from build123d import *

# Parameters (mm, degrees)
SKETCH1_W           = 20
SKETCH1_H           = 20
BOSS_EXTRUDE1_DEPTH = 20
SKETCH2_W           = 45
SKETCH2_H           = 70
BOSS_EXTRUDE2_DEPTH = 9
CUT_EXTRUDE1_DEPTH  = 5.8
FILLET1_R           = 3.6
FILLET2_R           = 10
SKETCH5_R           = 3.9
CUT_EXTRUDE2_DEPTH  = 51.717354032
CUT_EXTRUDE3_REACH  = 49.639
SKETCH6_R           = 1.75
SKETCH7_W           = 9
SKETCH7_H           = 45
CUT_EXTRUDE4_DEPTH  = 4.8
SKETCH9_W           = 9
SKETCH9_H           = 45
CUT_EXTRUDE5_DEPTH  = 23.8
SKETCH10_W          = 12.5
SKETCH10_H          = 41.4
CUT_EXTRUDE6_DEPTH  = 23.8
SKETCH11_W          = 20
SKETCH11_H          = 1.2
CUT_EXTRUDE7_DEPTH  = 23.8
BOSS_EXTRUDE3_START = 20
SKETCH12_W          = 20
SKETCH12_H          = 20
SKETCH12_R          = 3.9
BOSS_EXTRUDE3_DEPTH = 20
SKETCH13_W          = 20.2
SKETCH13_H          = 20.2
SKETCH13_R          = 3.9
BOSS_EXTRUDE4_DEPTH = 40
SKETCH14_W          = 9
SKETCH14_H          = 20
BOSS_EXTRUDE5_DEPTH = 0.1
SKETCH15_W          = 9
SKETCH15_H          = 40.3
BOSS_EXTRUDE6_DEPTH = 0.1
SKETCH16_W          = 9
SKETCH16_H          = 40.3
BOSS_EXTRUDE7_DEPTH = 0.1
SKETCH17_R          = 4.83091966
BOSS_EXTRUDE8_DEPTH = 39
SKETCH18_R          = 3
CUT_EXTRUDE8_DEPTH  = 2
FILLET3_R           = 3.23
FILLET4_R           = 4


# Some blends are built 0.0001 mm under size
with BuildPart() as part:
    # Sketch1 → Boss-Extrude1 (new body)
    with BuildSketch(Plane(origin=(0, 0, 0), x_dir=(0, 0, -1), z_dir=(1, 0, 0))):
        Rectangle(SKETCH1_W, SKETCH1_H)
    extrude(amount=BOSS_EXTRUDE1_DEPTH)

    # Sketch2 → Boss-Extrude2 (add)
    with BuildSketch(Plane(origin=(20, 0, 0), x_dir=(0, 0, -1), z_dir=(1, 0, 0))):
        Rectangle(SKETCH2_W, SKETCH2_H)
    extrude(amount=BOSS_EXTRUDE2_DEPTH)

    # Sketch4 → Cut-Extrude1 (cut)
    with BuildSketch(Plane(origin=(29, 0, 0), x_dir=(0, 0, -1), z_dir=(1, 0, 0))):
        with BuildLine():
            Line((3.6, -28.55), (-3.6, -28.55))
            Line((-3.6, -28.55), (-3.6, -7.311805523))
            ThreePointArc((-3.6, -7.311805523), (0, 8.15), (3.6, -7.311805523))
            Line((3.6, -7.311805523), (3.6, -28.55))
        make_face()
    extrude(amount=-CUT_EXTRUDE1_DEPTH, mode=Mode.SUBTRACT)

    # Fillet1
    fillet1_edges = [part.edges().sort_by_distance(p)[0] for p in [
        (26.1, -28.55, 3.6),
        (26.1, -28.55, -3.6),
    ]]
    fillet(fillet1_edges, radius=FILLET1_R - 0.0001)  # a hair under: the kernel refuses the full size

    # Fillet2
    fillet2_edges = [part.edges().sort_by_distance(p)[0] for p in [
        (26.1, -7.311805523, 3.6),
        (26.1, -7.311805523, -3.6),
    ]]
    fillet(fillet2_edges, radius=FILLET2_R)

    # Sketch5 → Cut-Extrude2 (cut, through all)
    with BuildSketch(Plane.ZY):
        Circle(SKETCH5_R)
    extrude(amount=-CUT_EXTRUDE2_DEPTH, mode=Mode.SUBTRACT)

    # Sketch6 → Cut-Extrude3 (cut, up to next)
    with BuildSketch(Plane(origin=(23.2, 0, 0), x_dir=(0, 0, -1), z_dir=(1, 0, 0)), mode=Mode.PRIVATE) as cut_extrude3_sk1:
        with Locations((0, -20.6)):
            Circle(SKETCH6_R)
    cut_extrude3_tool1 = extrude(cut_extrude3_sk1.sketch, amount=-CUT_EXTRUDE3_REACH, mode=Mode.PRIVATE) & part.part
    add(cut_extrude3_tool1.solids().sort_by_distance((23.2, -20.6, 0))[0], mode=Mode.SUBTRACT)

    # Sketch7 → Cut-Extrude4 (cut)
    with BuildSketch(Plane.XZ.offset(35)):
        with Locations((24.5, 0)):
            Rectangle(SKETCH7_W, SKETCH7_H)
    extrude(amount=-CUT_EXTRUDE4_DEPTH, mode=Mode.SUBTRACT)

    # Sketch9 → Cut-Extrude5 (cut)
    with BuildSketch(Plane(origin=(0, 35, 0), x_dir=(1, 0, 0), z_dir=(0, 1, 0))):
        with Locations((24.5, 0)):
            Rectangle(SKETCH9_W, SKETCH9_H)
    extrude(amount=-CUT_EXTRUDE5_DEPTH, mode=Mode.SUBTRACT)

    # Sketch10 → Cut-Extrude6 (cut)
    with BuildSketch(Plane.ZY.offset(-20)):
        with Locations((-16.25, -9.5)):
            Rectangle(SKETCH10_W, SKETCH10_H)
        with Locations((16.25, -9.5)):
            Rectangle(SKETCH10_W, SKETCH10_H)
    extrude(amount=-CUT_EXTRUDE6_DEPTH, mode=Mode.SUBTRACT)

    # Sketch11 → Cut-Extrude7 (cut)
    with BuildSketch(Plane.ZY.offset(-20)):
        with Locations((0, 10.6)):
            Rectangle(SKETCH11_W, SKETCH11_H)
    extrude(amount=-CUT_EXTRUDE7_DEPTH, mode=Mode.SUBTRACT)

    # Sketch12 → Boss-Extrude3 (add)
    with BuildSketch(Plane.ZY.offset(BOSS_EXTRUDE3_START)):
        Rectangle(SKETCH12_W, SKETCH12_H)
        Circle(SKETCH12_R, mode=Mode.SUBTRACT)
    extrude(amount=-BOSS_EXTRUDE3_DEPTH)

    # Sketch13 → Boss-Extrude4 (add)
    with BuildSketch(Plane.ZY.offset(20)):
        Rectangle(SKETCH13_W, SKETCH13_H)
        Circle(SKETCH13_R, mode=Mode.SUBTRACT)
    extrude(amount=-BOSS_EXTRUDE4_DEPTH)

    # Sketch14 → Boss-Extrude5 (add)
    with BuildSketch(Plane(origin=(0, 10, 0), x_dir=(1, 0, 0), z_dir=(0, 1, 0))):
        with Locations((24.5, 0)):
            Rectangle(SKETCH14_W, SKETCH14_H)
    extrude(amount=BOSS_EXTRUDE5_DEPTH)

    # Sketch15 → Boss-Extrude6 (add)
    with BuildSketch(Plane.XY.offset(10)):
        with Locations((24.5, -10.05)):
            Rectangle(SKETCH15_W, SKETCH15_H)
    extrude(amount=BOSS_EXTRUDE6_DEPTH)

    # Sketch16 → Boss-Extrude7 (add)
    with BuildSketch(Plane(origin=(0, 0, -10), x_dir=(-1, 0, 0), z_dir=(0, 0, -1))):
        with Locations((-24.5, -10.05)):
            Rectangle(SKETCH16_W, SKETCH16_H)
    extrude(amount=BOSS_EXTRUDE7_DEPTH)

    # Sketch17 → Boss-Extrude8 (add)
    with BuildSketch(Plane.ZY.offset(20)):
        Circle(SKETCH17_R)
    extrude(amount=-BOSS_EXTRUDE8_DEPTH)

    # Sketch18 → Cut-Extrude8 (cut)
    with BuildSketch(Plane.ZY.offset(20)):
        Circle(SKETCH18_R)
    extrude(amount=-CUT_EXTRUDE8_DEPTH, mode=Mode.SUBTRACT)

    # Fillet3
    # the kernel refuses this fillet: 3.23 mm, written as the material it adds along each edge
    with BuildSketch(Plane(origin=(-18, 0, 0), x_dir=(0, 0, 1), z_dir=(0, -1, 0))) as fillet3_piece_1:
        with BuildLine():
            CenterArc((0.013363095, 3.23), FILLET3_R, 270, 67.616447755)
            Line((0.013363095, 0), (0.013363095, -0.0646))
            Line((0.013363095, -0.0646), (3, -0.0646))
            Line((3, -0.0646), (3.0646, 0))
            ThreePointArc((3.0646, 0), (3.0646, 1), (3.059732738, 1.9754))
            Line((3.059732738, 1.9754), (3, 2))
        make_face()
    revolve(axis=Axis((-18, 0, 0), (-1, 0, 0)))

    # Fillet4
    fillet4_edges = [part.edges().sort_by_distance(p)[0] for p in [
        (24.5, -30.2, 10.1),
        (24.5, -30.2, -10.1),
    ]]
    fillet(fillet4_edges, radius=FILLET4_R)


solid = part.part
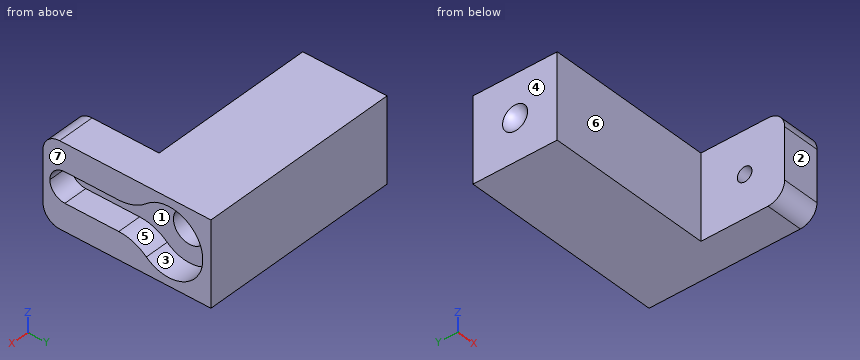
Work out the finished part from the listing and answer in its coordinate system (mm). Face numbers are marked on the shaded views. A direction names the side the tool comes from. Give positions to 0.01 mm unless a question says otherwise; leave off trailing zeros. Write each loop counter-clockwise with the first axis right and the second up, starting at its lowest first coordinate (ties: lowest second). Pieces come first, ordered by that corner, then holes.
Q1. The part is cut by section B-B on z = 7. Give the vertices of the cut face in (x, y).
Answer:
outline: (-20, -10.1) - (20, -10.1) - (20, -30.1) - (29, -30.1) - (29, -4.17) - (23.2, -4.17) - (23.2, 4.17) - (29, 4.17) - (29, 10.1) - (-20, 10.1) - close
Q2. For a pull along Y with two mould halves and no side action, classify the marked faces 1, 2, 3 and 4 as released by +Y, released by -Y, zero draft, split by the parting line, or undercut.
Answer:
face 1: undercut
face 2: released by -Y
face 3: undercut
face 4: zero draft
Q3. The part is cut by section C-C on x = 15.5. Give the vertices of the cut face in (y, z), and give its area (3 significant figures).
Answer:
outline: (-10.1, -10.1) - (10.1, -10.1) - (10.1, 10.1) - (-10.1, 10.1) - close
area: 408 mm2
Q4. Straight lines are drawn through the part: L1, parallel to Y at x = 21.85, z = 0; L2, parallel to Y at x = 26.05, z = 0; L3, parallel to Z at x = 24.4, y = 0. For each, find the intervals that lie inside material, in ascending order.
Answer:
L1: y = -30.2 to -22.35, -18.85 to -3.9, 3.9 to 10.1
L2: y = -30.2 to -28.55, 8.15 to 10.1
L3: z = -10.1 to -8.15, 8.15 to 10.1
Q5. A tool of negligible diameter and unlimited length cuts with its end or side. For the marked faces 5, 6 and 7, from which of +Z, -Z, +X, -X, +Y, -Y can it reach the whole face along a straight path? Write none if from no direction.
Answer:
face 5: +X
face 6: +Z, -Z, -X, -Y
face 7: +Z, -Z, +X, +Y, -Y
Q6. Given pin 1 (6 mm diameter, centred on x = 8, z = -8, fed in from -Y); pin 2 (4 mm diameter, centred on y = -0.5, z = -0.5, fed in from +X), each flat-ended and moving along its own axis, determine where each tip first touches the part or whether it passes through.
Answer:
pin 1: stops at y = -10.1
pin 2: stops at x = 19
Q7. The part is cut by section A-A on y = -20.6. Give the vertices of the cut face in (x, z), and give its area (3 significant figures).
Answer:
outline: (20, -10.1) - (29, -10.1) - (29, -3.6) - (23.2, -3.6) - (23.2, -1.75) - (20, -1.75) - close; (20, 1.75) - (23.2, 1.75) - (23.2, 3.6) - (29, 3.6) - (29, 10.1) - (20, 10.1) - close
area: 129 mm2
